Verification items for this drawing (mm, ordinates from the low corner). Coordinates: 2 decimals unless noted, no trailing zeros. Order: outer loops, then holes, each group sorted by start corner. A loop starts at its lowest first (then second) coordinate and runs counter-clockwise, first axis right, second up.
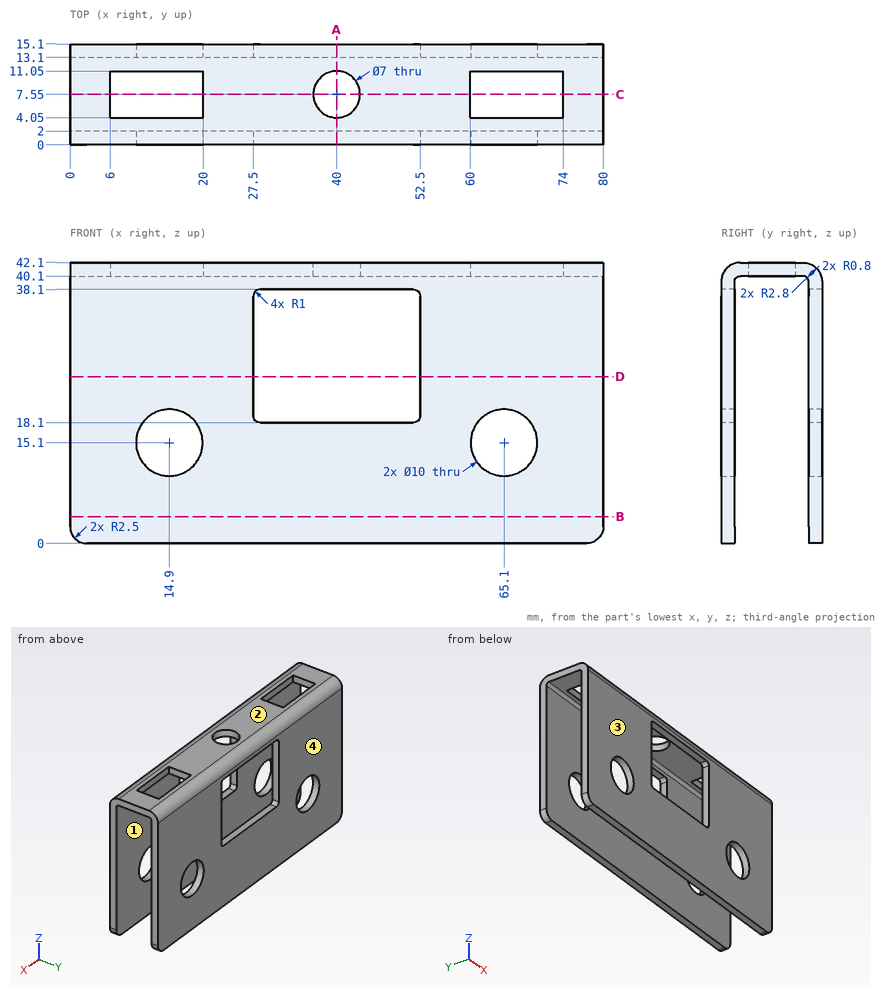
Item 1: Depth check by flat-ended pin: P1, Ø6.5, axis at x = 40, y = 7.55, coming from the -Z side; P2, Ø4, axis at x = 70.5, y = 5.5, coming from the -Z side; P3, Ø1.5, axis at x = 13.5, y = 13.5, coming from the +Z side; P4, Ø1, axis at x = 65, z = 41, coming from the +Y side. Enter the tip coordinate at first touch or a pass-through.
Item 2: Thickness scan on line 1 along X through (y, z) = (14.5, 15.1); line 2 along Y through (x, z) = (74, 5); line 3 along Z through (x, y) = (46.5, 0.75). Record the ranges inside material, lowest first.
Item 3: Sectioned sample at A-A (x = 40). Record the cut outline in (y, z), and give its area (3 significant figures).
Item 4: Sectioned sample at C-C (y = 7.55). Record the cut outline in (x, z).
Item 5: Sectioned sample at B-B (z = 4). Record the cut outline in (x, y).
Item 6: Sectioned sample at D-D (z = 25). Record the cut outline in (x, y).
Item 7: Release check for a two-part mould opening along Y. For the marked faces 1, 2, 3 and 4 record: pulls with the +Y half, pulls with the -Y half, needs draft (parallel to the pull), parting line crosses it, or undercut.
Geometry check:
1. P1: passes through
1. P2: stops at z = 40.1
1. P3: stops at z = 42.06
1. P4: stops at y = 14.83
2. line 1: x = 0 to 9.9, 19.9 to 60.1, 70.1 to 80
2. line 2: y = 0 to 2, 13.1 to 15.1
2. line 3: z = 0 to 18.1, 38.1 to 41.21
3. outline: (0, 0) - (2, 0) - (2, 18.1) - (0, 18.1) - close; (0, 38.1) - (2, 38.1) - (2, 39.3) arc R0.8 cw to (2.8, 40.1) - (4.05, 40.1) - (4.05, 42.1) - (2.8, 42.1) arc R2.8 ccw to (0, 39.3) - close; (11.05, 40.1) - (12.3, 40.1) arc R0.8 cw to (13.1, 39.3) - (13.1, 38.1) - (15.1, 38.1) - (15.1, 39.3) arc R2.8 ccw to (12.3, 42.1) - (11.05, 42.1) - close; (13.1, 0) - (15.1, 0) - (15.1, 18.1) - (13.1, 18.1) - close
3. area: 93.5 mm2
4. outline: (0, 40.1) - (6, 40.1) - (6, 42.1) - (0, 42.1) - close; (20, 40.1) - (36.5, 40.1) - (36.5, 42.1) - (20, 42.1) - close; (43.5, 40.1) - (60, 40.1) - (60, 42.1) - (43.5, 42.1) - close; (74, 40.1) - (80, 40.1) - (80, 42.1) - (74, 42.1) - close
5. outline: (0, 0) - (80, 0) - (80, 2) - (0, 2) - close; (0, 13.1) - (80, 13.1) - (80, 15.1) - (0, 15.1) - close
6. outline: (0, 0) - (27.5, 0) - (27.5, 2) - (0, 2) - close; (0, 13.1) - (27.5, 13.1) - (27.5, 15.1) - (0, 15.1) - close; (52.5, 0) - (80, 0) - (80, 2) - (52.5, 2) - close; (52.5, 13.1) - (80, 13.1) - (80, 15.1) - (52.5, 15.1) - close
7. face 1: undercut
7. face 2: needs draft
7. face 3: pulls with the -Y half
7. face 4: pulls with the +Y half
